Here's how the part is built. I have some questions about the finished solid (model axes, mm). Round coordinates to 2 decimals unless told otherwise and drop trailing zeros. Order: outer loops, then holes, each group sorted by start corner. A loop starts at its lowest first (then second) coordinate and runs counter-clockwise, first axis right, second up. Notation, with made-up numbers: (47, 83.25) - (78, 83.25) arc R17 ccw to (78, 102.25) - close; hole circle Ø11 at (41.25, 75). An arc over 180 degrees is marked (long way). Answer as a JSON object with one key per item and string values.
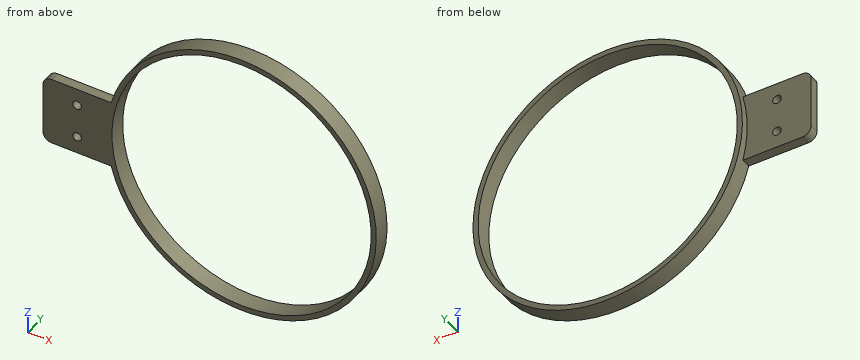
```python
from build123d import *

# Parameters (mm, degrees)
CROQUIS1_R              = 79
CROQUIS1_R_2            = 76
SALIENTE_EXTRUIR1_DEPTH = 10
CROQUIS2_R              = 2.499891185
CROQUIS2_R_2            = 2.5
SALIENTE_EXTRUIR2_DEPTH = 5.5


with BuildPart() as part:
    # Croquis1 → Saliente-Extruir1 (new body)
    with BuildSketch(Plane(origin=(0, 0, 0), x_dir=(1, 0, 0), z_dir=(0, 1, 0))):
        with Locations(Location((0, 0, 0), (0, 0, 270))):
            Circle(CROQUIS1_R)
        with Locations(Location((0, 0, 0), (0, 0, 270))):
            Circle(CROQUIS1_R_2, mode=Mode.SUBTRACT)
    extrude(amount=SALIENTE_EXTRUIR1_DEPTH)

    # Croquis2 → Saliente-Extruir2 (add)
    with BuildSketch(Plane(origin=(0, 0, 0), x_dir=(1, 0, 0), z_dir=(0, 1, 0))):
        with BuildLine():
            Line((-76.426435217, 20), (-111.426435217, 20))
            ThreePointArc((-111.426435217, 20), (-114.961969123, 18.535533906), (-116.426435217, 15))
            Line((-116.426435217, 15), (-116.426435217, -15))
            ThreePointArc((-116.426435217, -15), (-114.961969123, -18.535533906), (-111.426435217, -20))
            Line((-111.426435217, -20), (-76.426435217, -20))
            ThreePointArc((-76.426435217, -20), (-79, 0), (-76.426435217, 20))
        make_face()
        with Locations(Location((-96.426435217, 10, 0), (0, 0, 270))):
            Circle(CROQUIS2_R, mode=Mode.SUBTRACT)
        with Locations(Location((-96.426435217, -10, 0), (0, 0, 270))):
            Circle(CROQUIS2_R_2, mode=Mode.SUBTRACT)
    extrude(amount=SALIENTE_EXTRUIR2_DEPTH)


solid = part.part
```
1. Imagine slicing it at C-C (z = -10). List the corners of the cut face in (x, y) for me.
Responses:
{"outline": "(-116.43, 0) - (-98.93, 0) - (-98.93, 5.5) - (-116.43, 5.5) - close; (-93.93, 0) - (-75.34, 0) - (-75.34, 10) - (-78.36, 10) - (-78.36, 5.5) - (-93.93, 5.5) - close; (75.34, 0) - (78.36, 0) - (78.36, 10) - (75.34, 10) - close"}
2. Imagine slicing it at A-A (x = 0). List the corners of the cut face in (y, z) for me.
Responses:
{"outline": "(0, -79) - (10, -79) - (10, -76) - (0, -76) - close; (0, 76) - (10, 76) - (10, 79) - (0, 79) - close"}
3. If I drill on L1, parallel to X at y = 2.6, z = -10; L2, parallel to Z at x = -2, y = 5.75; L3, parallel to X at y = 3.75, z = 0, over which ranges is the centre line in solid material (lowest first)? Write a range as [from, to].
Responses:
{"L1": "[-116.43, -98.93], [-93.93, -75.34], [75.34, 78.36]", "L2": "[-78.97, -75.97], [75.97, 78.97]", "L3": "[-116.43, -76], [76, 79]"}
4. Imagine slicing it at D-D (y = 2.75). List the corners of the cut face in (x, z) for me.
Responses:
{"outline": "(-116.43, -15) arc R5 ccw to (-111.43, -20) - (-76.43, -20) arc R79 ccw (long way) to (-76.43, 20) - (-111.43, 20) arc R5 ccw to (-116.43, 15) - close; hole circle Ø5 at (-96.43, -10); hole circle Ø5 at (-96.43, 10); hole circle Ø152 at (0, 0)"}
5. For P1, Ø1.5, axis at x = 29.5, y = 2.5, coming from the -Z side; P2, Ø5, axis at x = 45.5, z = 58, coming from the +Y side; P3, Ø3, axis at y = 4, z = -42.5, coming from the -X side; P4, Ø6, axis at x = -32.5, y = 7, coming from the -Z side, each with a flat end and sliding along its axis, tell me the tip position at first contact or that it passes through.
Responses:
{"P1": "z = -73.58", "P2": "y = 10", "P3": "x = -67.53", "P4": "z = -73.29"}
6. Imagine slicing it at B-B (z = -58.5). List the corners of the cut face in (x, y) for me, plus the area to 3 significant figures.
Responses:
{"outline": "(-53.09, 0) - (-48.52, 0) - (-48.52, 10) - (-53.09, 10) - close; (48.52, 0) - (53.09, 0) - (53.09, 10) - (48.52, 10) - close", "area": "91.5 mm2"}
